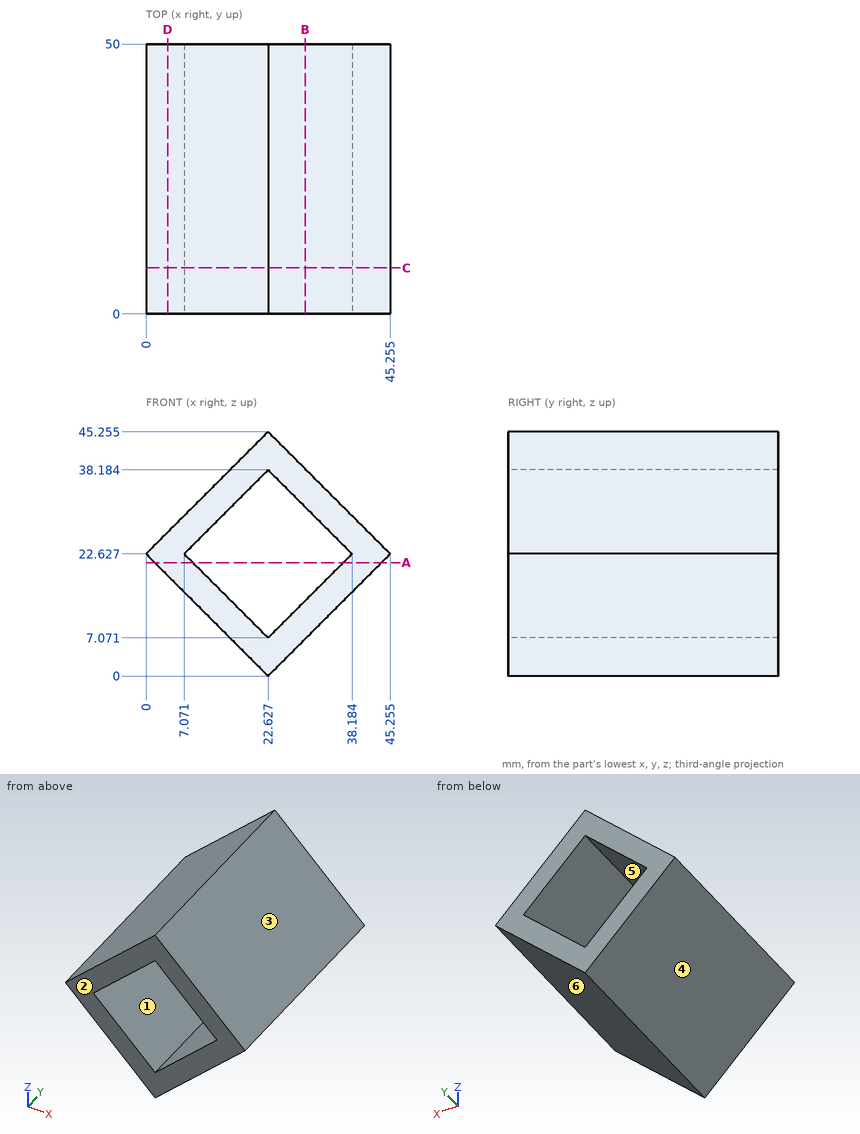
The drawing under review shows one solid part. Ordinate dimensions are in mm from its lowest x, y, z. A direction names the side the tool comes from. Give positions to 0.01 mm unless a question says otherwise; leave off trailing zeros. Order: outer loops, then holes, each group sorted by start corner. A loop starts at its lowest first (then second) coordinate and runs counter-clockwise, first axis right, second up. Notation, with made-up numbers: (81, -9.75) -> (87, -9.75) arc R21 ccw to (87, 24.25) -> close; hole circle Ø6 at (47.25, 6.25). An arc over 180 degrees is marked (long way). Write item = value, one per line.
1) Insertion check: pin 1 (3 mm diameter, centred on y = 22, z = 25.5, fed in from +X); pin 2 (5 mm diameter, centred on x = 20.5, y = 22.5, fed in from -Z); pin 3 (4 mm diameter, centred on y = 43.5, z = 33.5, fed in from +X); pin 4 (3 mm diameter, centred on x = 28.5, z = 9, fed in from -Y). Each pin has a flat end and moves straight along its axis. Give the tip position at first contact, or say it passes through.
Findings:
pin_1 = 43.88
pin_2 = 0
pin_3 = 36.38
pin_4 = 0
2) Draft analysis for pull direction X (two halves, no side actions). For the marked faces 1, 2, 3 and 4, state which applies: pulls with the +X half, pulls with the -X half, needs draft (parallel to the pull), parting line crosses it, or undercut.
Findings:
face_1 = undercut
face_2 = needs draft
face_3 = pulls with the +X half
face_4 = pulls with the -X half
3) To check wall thickness, follow L1, parallel to X at y = 14, z = 32 (1 decimal); L2, parallel to X at y = 35, z = 20 (1 decimal); L3, parallel to Z at x = 17, y = 4 (1 decimal). State the ranges of each line that lie inside material, in increasing order. Write a range as from..to.
Findings:
L1 = 9.4..16.4, 28.8..35.9
L2 = 2.6..9.7, 35.6..42.6
L3 = 5.6..12.7, 32.6..39.6
4) We need section C-C, the plane y = 8.5. Give the boundary of the cut face in (x, z) (1 decimal), and give its area (3 significant figures).
Findings:
outline = (0, 22.6) -> (22.6, 0) -> (45.3, 22.6) -> (22.6, 45.3) -> close; hole (7.1, 22.6) -> (22.6, 7.1) -> (38.2, 22.6) -> (22.6, 38.2) -> close
area = 540 mm^2
5) We need section A-A, the plane z = 21. Give the boundary of the cut face in (x, y), and give its area (3 significant figures).
Findings:
outline = (1.63, 0) -> (8.7, 0) -> (8.7, 50) -> (1.63, 50) -> close; (36.56, 0) -> (43.63, 0) -> (43.63, 50) -> (36.56, 50) -> close
area = 707 mm^2
6) We need section D-D, the plane x = 4. Give the boundary of the cut face in (y, z), and give its area (3 significant figures).
Findings:
outline = (0, 18.63) -> (50, 18.63) -> (50, 26.63) -> (0, 26.63) -> close
area = 400 mm^2
7) For the marked faces 5 and 6, list the 3-axis set-ups (+Z, -Z, +X, -X, +Y, -Y) from which the entire face can be reached by the end or side of a thin tool; tool diameter is ignored.
Findings:
face_5 = +Y, -Y
face_6 = -Z, +X, +Y, -Y
8) We need section B-B, the plane x = 29.5. Give the boundary of the cut face in (y, z), and give its area (3 significant figures).
Findings:
outline = (0, 6.87) -> (50, 6.87) -> (50, 13.94) -> (0, 13.94) -> close; (0, 31.31) -> (50, 31.31) -> (50, 38.38) -> (0, 38.38) -> close
area = 707 mm^2
